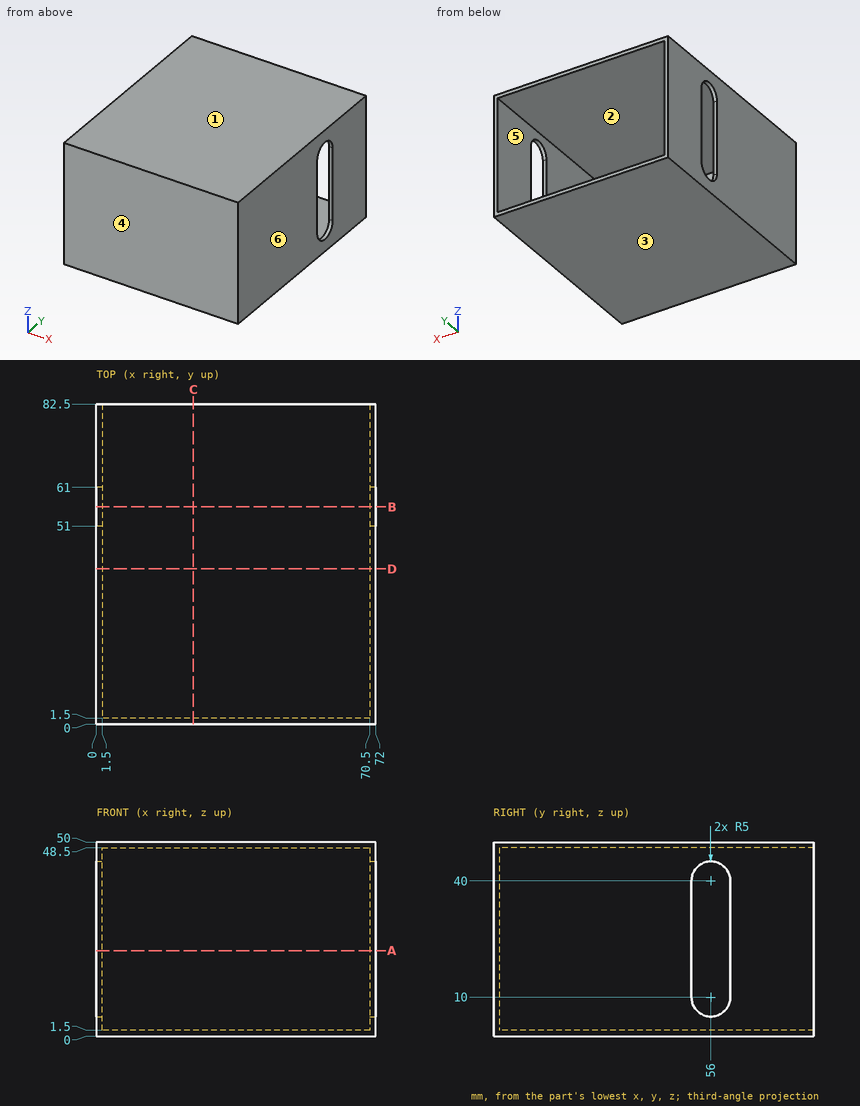
Here's the drawing with two shaded views (mm, measured from the low corner). I have some questions. A direction names the side the tool comes from. Coordinates: 2 decimals unless noted, no trailing zeros. Write each loop counter-clockwise with the first axis right and the second up, starting at its lowest first coordinate (ties: lowest second). Pieces come first, ordered by that corner, then holes. Notation, with made-up numbers: (52.25, 41.5) - (80.25, 41.5) arc R26 cw to (80.25, 70.5) - close; hole circle Ø10 at (48.5, 76). An arc over 180 degrees is marked (long way). Return JSON: item names as keys, results as strings.
Q1. If we section it at C-C (x = 25): Please give me the cut outline in (y, z).
Computed values:
{"outline": "(0, 0) - (82.5, 0) - (82.5, 1.5) - (1.5, 1.5) - (1.5, 48.5) - (82.5, 48.5) - (82.5, 50) - (0, 50) - close"}
Q2. Please list where these lines run through material, in increasing order: L1, parallel to Z at x = 11, y = 12; L2, parallel to X at y = 46.5, z = 13; L3, parallel to Y at x = 15.5, z = 12. Write a range as from..to.
Computed values:
{"L1": "z = 0..1.5, 48.5..50", "L2": "x = 0..1.5, 70.5..72", "L3": "y = 0..1.5"}
Q3. If we section it at D-D (y = 40): Please give me the cut outline in (x, z), then the cut area to 3 significant figures.
Computed values:
{"outline": "(0, 0) - (72, 0) - (72, 50) - (0, 50) - close; hole (1.5, 1.5) - (70.5, 1.5) - (70.5, 48.5) - (1.5, 48.5) - close", "area": "357 mm2"}
Q4. Thinking about a two-plate mould opening in Z: for the marked faces 1, 2, 3 and 4, which applies, +Z half, -Z half, draft (parallel to the pull), parting line (faces both ways), or undercut?
Computed values:
{"face 1": "+Z half", "face 2": "undercut", "face 3": "-Z half", "face 4": "draft"}
Q5. On a 3-axis mill with a long thin cutter (end or side, diameter ignored), from which of +Z, -Z, +X, -X, +Y, -Y can I reach the whole of each face in a straight line? I mean the marked faces 5 and 6. Say none if no direction works.
Computed values:
{"face 5": "+Y", "face 6": "+Z, -Z, +X, +Y, -Y"}
Q6. If we section it at B-B (y = 56): Please give me the cut outline in (x, z), then the cut area to 3 significant figures.
Computed values:
{"outline": "(0, 0) - (72, 0) - (72, 5) - (70.5, 5) - (70.5, 1.5) - (1.5, 1.5) - (1.5, 5) - (0, 5) - close; (0, 45) - (1.5, 45) - (1.5, 48.5) - (70.5, 48.5) - (70.5, 45) - (72, 45) - (72, 50) - (0, 50) - close", "area": "237 mm2"}
Q7. If we section it at A-A (z = 22): Please give me the cut outline in (x, y).
Computed values:
{"outline": "(0, 0) - (72, 0) - (72, 51) - (70.5, 51) - (70.5, 1.5) - (1.5, 1.5) - (1.5, 51) - (0, 51) - close; (0, 61) - (1.5, 61) - (1.5, 82.5) - (0, 82.5) - close; (70.5, 61) - (72, 61) - (72, 82.5) - (70.5, 82.5) - close"}
